```python
from build123d import *

# Parameters (mm, degrees)
SCHIZZO2_R                   = 2
SCHIZZO2_R_2                 = 1.343240654
ESTRUSIONE_ESTRUSIONE1_DEPTH = 15
SCHIZZO3_R                   = 7.5
TAGLIO_ESTRUSIONE1_DEPTH     = 11
SMUSSO3_SIZE                 = 1
RACCORDO1_R                  = 2.5
SMUSSO4_SIZE                 = 4
SMUSSO4_SIZE2                = 2.800830153
TAGLIO_ESTRUSIONE3_DEPTH     = 46.276925691
FILLET1_R                    = 5
FILLET3_R                    = 5
FILLET4_R                    = 5
FILLET5_R                    = 5
SKETCH1_R                    = 3
CUT_EXTRUDE1_DEPTH           = 5


with BuildPart() as part:
    # Schizzo2 → Estrusione-Estrusione1 (new body)
    with BuildSketch(Plane.XY):
        Polygon((-40, 0), (-2, 0), (0.321661039, 2.321661039), (0.321661039, 9), (-7.024563842, 9), (-14.880083854, 15), (-23.119916146, 15), (-30.975436158, 9), (-40, 9), align=None)
        with Locations((-19, 10)):
            Circle(SCHIZZO2_R, mode=Mode.SUBTRACT)
        with Locations((-3.5, 5.5)):
            Circle(SCHIZZO2_R_2, mode=Mode.SUBTRACT)
    extrude(amount=-ESTRUSIONE_ESTRUSIONE1_DEPTH)

    # Schizzo3 → Taglio-Estrusione1 (cut)
    with BuildSketch(Plane(origin=(0, 0, -15), x_dir=(-1, 0, 0), z_dir=(0, 0, -1))):
        with Locations((19, 10)):
            Circle(SCHIZZO3_R)
    extrude(amount=-TAGLIO_ESTRUSIONE1_DEPTH, mode=Mode.SUBTRACT)

    # Smusso3
    # the kernel refuses this chamfer: 1, 0.730975935 mm, written as the material it takes off along each edge
    with BuildSketch(Plane(origin=(-25.938580935, 12.847120406, -4), x_dir=(-0.7947073367402627, -0.6069927914985472, 0), z_dir=(0, 0, -1))) as smusso3_piece_1:
        with BuildLine():
            Line((SMUSSO3_SIZE, 0), (0.605555486, -0.394444514))
            ThreePointArc((0.605555486, -0.394444514), (0.30405624, -0.187661825), (0, 0))
            Line((0, 0), (SMUSSO3_SIZE, 0))
        make_face()
    extrude(amount=13.571682988, mode=Mode.SUBTRACT)
    with BuildSketch(Plane(origin=(-12.061419065, 12.847120406, -4), x_dir=(0.33460224521765425, -0.94235945238285, 0), z_dir=(0, 0, -1))) as smusso3_piece_2:
        with BuildLine():
            Line((0.722692134, 0), (SMUSSO3_SIZE * 0.837916253761, -SMUSSO3_SIZE * 0.545798819789))
            Line((SMUSSO3_SIZE * 0.837916253761, -SMUSSO3_SIZE * 0.545798819789), (0, 0))
            ThreePointArc((0, 0), (0.357199268, -0.008708643), (0.722692134, 0))
        make_face()
    extrude(amount=13.571682988, mode=Mode.SUBTRACT)

    # Raccordo1
    raccordo1_edges = [part.edges().sort_by_distance(p)[0] for p in [
        (0.321661039, 9, -7.5),
    ]]
    fillet(raccordo1_edges, radius=RACCORDO1_R)

    # Smusso4
    smusso4_edges = [part.edges().sort_by_distance(p)[0] for p in [
        (-40, 9, -7.5),
    ]]
    smusso4_side = [part.faces().sort_by_distance(p)[0] for p in [
        (-40, 4.5, -7.5),
    ]]
    chamfer(smusso4_edges, length=SMUSSO4_SIZE, length2=SMUSSO4_SIZE2, reference=smusso4_side[0])

    # Schizzo5 → Taglio-Estrusione3 (cut, through all)
    with BuildSketch(Plane.XZ):
        with BuildLine():
            Line((-35.611900304, -3), (-32.611900304, -3))
            ThreePointArc((-32.611900304, -3), (-30.611900304, -5), (-32.611900304, -7))
            Line((-32.611900304, -7), (-35.611900304, -7))
            ThreePointArc((-35.611900304, -7), (-37.611900304, -5), (-35.611900304, -3))
        make_face()
    extrude(amount=-TAGLIO_ESTRUSIONE3_DEPTH, mode=Mode.SUBTRACT)

    # Fillet1
    fillet1_edges = [part.edges().sort_by_distance(p)[0] for p in [
        (-7.024563842, 9, -7.5),
    ]]
    fillet(fillet1_edges, radius=FILLET1_R)

    # Fillet3
    # the kernel refuses this fillet: 5 mm, written as the material it takes off along each edge
    with BuildSketch(Plane(origin=(-37.199169847, 9, 0.290299162), x_dir=(-0.573576436351049, -0.8191520442889898, 0), z_dir=(0, 0, -1))) as fillet3_piece_1:
        with BuildLine():
            CenterArc((FILLET3_R * 0.520567050552, -FILLET3_R), FILLET3_R, 90, 55)
            Line((-FILLET3_R * 0.298584993737, -FILLET3_R * 0.426423563649), (0, 0))
            Line((0, 0), (FILLET3_R * 0.520567050552, 0))
        make_face()
    extrude(amount=21.797387294, mode=Mode.SUBTRACT)
    with BuildSketch(Plane(origin=(-40, 5, 3.941234861), x_dir=(0, -1, 0), z_dir=(0, 0, -1))) as fillet3_piece_2:
        with BuildLine():
            CenterArc((FILLET3_R * 0.315298788879, -FILLET3_R), FILLET3_R, 90, 35)
            Line((-FILLET3_R * 0.258277647472, -FILLET3_R * 0.180847955711), (0, 0))
            Line((0, 0), (FILLET3_R * 0.315298788879, 0))
        make_face()
    extrude(amount=22.882469722, mode=Mode.SUBTRACT)
    with BuildSketch(Plane(origin=(-37.199169847, 9, 6.507088132), x_dir=(-0.573576436351049, -0.8191520442889898, 0), z_dir=(0, 0, -1))) as fillet3_piece_3:
        with BuildLine():
            CenterArc((FILLET3_R * 0.520567050552, -FILLET3_R), FILLET3_R, 90, 55)
            Line((-FILLET3_R * 0.298584993737, -FILLET3_R * 0.426423563649), (0, 0))
            Line((0, 0), (FILLET3_R * 0.520567050552, 0))
        make_face()
    extrude(amount=16.797387294, mode=Mode.SUBTRACT)

    # Fillet4
    fillet4_edges = [part.edges().sort_by_distance(p)[0] for p in [
        (-14.880083854, 15, -2),
        (-23.119916146, 15, -2),
    ]]
    fillet(fillet4_edges, radius=FILLET4_R)

    # Fillet5
    # the kernel refuses this fillet: 5 mm, written as the material it adds along each edge
    with BuildSketch(Plane(origin=(-30.975436158, 9, -1.922117515), x_dir=(0.794707336740263, 0.6069927914985467, 0), z_dir=(0, 0, -1))) as fillet5_piece_1_section:
        with BuildLine():
            CenterArc((FILLET5_R * 0.338212687424, -FILLET5_R), FILLET5_R, 90, 37.372378399)
            Line((-FILLET5_R * 0.268780104075, -FILLET5_R * 0.20529266326), (0, 0))
            Line((0, 0), (FILLET5_R * 0.338212687424, 0))
        make_face()
    fillet5_piece_1 = extrude(amount=13.077882485, mode=Mode.PRIVATE)
    fillet5_piece_1 = fillet5_piece_1 - Plane(origin=(-32.611900304, 9, -5), x_dir=(0, 0, 1), z_dir=(0, -1, 0)) * Cylinder(2, 33, mode=Mode.PRIVATE)
    add(fillet5_piece_1)
    with BuildSketch(Plane(origin=(-30.975436158, 9, 0), x_dir=(0.794707336740263, 0.6069927914985467, 0), z_dir=(0, 0, -1))) as fillet5_piece_2_section:
        with BuildLine():
            CenterArc((FILLET5_R * 0.338212687424, -FILLET5_R), FILLET5_R, 90, 37.372378399)
            Line((-FILLET5_R * 0.268780104075, -FILLET5_R * 0.20529266326), (0, 0))
            Line((0, 0), (FILLET5_R * 0.338212687424, 0))
        make_face()
    fillet5_piece_2 = extrude(amount=8.077882485, mode=Mode.PRIVATE)
    fillet5_piece_2 = fillet5_piece_2 - Plane(origin=(-32.611900304, 9, -5), x_dir=(0, 0, 1), z_dir=(0, -1, 0)) * Cylinder(2, 23, mode=Mode.PRIVATE)
    add(fillet5_piece_2)

    # Sketch1 → Cut-Extrude1 (cut)
    with BuildSketch(Plane.XY):
        with Locations((-3.5, 5.5)):
            Circle(SKETCH1_R)
    extrude(amount=-CUT_EXTRUDE1_DEPTH, mode=Mode.SUBTRACT)


solid = part.part
```
Here's how the part is built. I have some questions about the finished solid (model axes, mm). A direction names the side the tool comes from. Round coordinates to 2 decimals unless told otherwise and drop trailing zeros. Loops run counter-clockwise (first coordinate to the right, second up) from the corner with the lowest first, then second, coordinate; pieces in that order, holes last.
1. Suppose I cut it at D-D, the plane y = 11.25. Please give me the cut outline in (x, z).
Answers:
outline: (-28.03, -15) - (-26.4, -15) - (-26.4, -4) - (-20.56, -4) - (-20.56, 0) - (-28.03, 0) - close; (-17.44, -4) - (-11.6, -4) - (-11.6, -15) - (-9.97, -15) - (-9.97, 0) - (-17.44, 0) - close
2. Suppose I cut it at A-A, the plane z = -6. Please give me the cut outline in (x, y).
Answers:
outline: (-40, 0) - (-37.34, 0) - (-37.34, 8.18) arc R5 ccw to (-38.69, 6.87) - (-39.1, 6.29) arc R5 ccw to (-40, 3.42) - close; (-30.88, 0) - (-2, 0) - (0.32, 2.32) - (0.32, 6.5) arc R2.5 ccw to (-2.18, 9) - (-5.33, 9) arc R5 cw to (-8.37, 10.03) - (-11.27, 12.24) - (-11.82, 12.17) arc R7.5 cw (long way) to (-26.18, 12.17) - (-26.73, 12.24) - (-29.63, 10.03) arc R5 cw to (-30.88, 9.33) - close; hole circle Ø2.69 at (-3.5, 5.5)
3. Will these pins go through, and if not, where does the flat tip stop? pin 1 (0.6 mm diameter, centred on x = -33.5, z = -1, fed in from +Y); pin 2 (5 mm diameter, centred on x = -19, y = 10, fed in from -Z); pin 3 (1.5 mm diameter, centred on y = 11, z = -9, fed in from +X); pin 4 (2 mm diameter, centred on x = -3.5, y = 5.5, fed in from +Z).
Answers:
pin 1: stops at y = 9
pin 2: stops at z = -4
pin 3: stops at x = -8.66
pin 4: passes through
4. If I drill on probe 1 along Y at (x, z) = (-3.5, -1.9); probe 2 along Z at (x, y) = (-34.5, 3.25); probe 3 along Y at (x, z) = (-19, -2.9), over which ranges is the centre line in solid material (lowest first)?
Answers:
probe 1: y = 0 to 2.5, 8.5 to 9
probe 2: z = -15 to -7, -3 to 0
probe 3: y = 0 to 8, 12 to 15
5. Suppose I cut it at C-C, the plane z = -11.5. Please give me the cut outline in (x, y), and give its area (3 significant figures).
Answers:
outline: (-40, 0) - (-2, 0) - (0.32, 2.32) - (0.32, 6.5) arc R2.5 ccw to (-2.18, 9) - (-5.33, 9) arc R5 cw to (-8.37, 10.03) - (-11.27, 12.24) - (-11.82, 12.17) arc R7.5 cw (long way) to (-26.18, 12.17) - (-26.73, 12.24) - (-29.63, 10.03) arc R5 cw to (-32.67, 9) - (-34.6, 9) arc R5 ccw to (-38.69, 6.87) - (-39.1, 6.29) arc R5 ccw to (-40, 3.42) - close; hole circle Ø2.69 at (-3.5, 5.5)
area: 289 mm2
6. Suppose I cut it at B-B, the plane x = -34. Please give me the cut outline in (y, z), and give its area (3 significant figures).
Answers:
outline: (0, -15) - (9, -15) - (9, -7) - (0, -7) - close; (0, -3) - (9, -3) - (9, 0) - (0, 0) - close
area: 99.0 mm2
7. For faces 1 (the face through (-30.612, 4.655, -5.045)), 2 (the face through (-34, 9, -1)), 3 (the face through (-4, 9, -7)), which set-ups out of +Z, -Z, +X, -X, +Y, -Y let a thin tool reach every point of the face, with its end or its side?
Answers:
face 1: +Y, -Y
face 2: +Z, -Z, -X, +Y
face 3: +Z, -Z, +X, +Y
8. Thinking about a two-plate mould opening in Z: for faces 4 (the face through (-34, 4, -7)), 5 (the face through (-23.009, 14.744, -2.028)), 6 (the face through (-19, 2, -15)), which applies, released by +Z, released by -Z, zero draft, split by the parting line, or undercut?
Answers:
face 4: undercut
face 5: zero draft
face 6: released by -Z
